Solid Edge part; units mm, degrees
sketch "Sketch1" plane through (0, 0, 0) normal (0, 0, 1) x (1, 0, 0)
  circle A0 centre (0, 0) radius 8
extrude "Protrusion1" add sketch "Sketch1" along normal blind 10
sketch "Sketch2" plane through (0, 0, 0) normal (0, 0, -1) x (1, 0, 0)
  circle A0 centre (0, 0) radius 5
extrude "Protrusion2" add sketch "Sketch2" along normal blind 55
sketch "Sketch3" plane through (0, 0, -55) normal (0, 0, -1) x (1, 0, 0)
  circle A0 centre (0, 0) radius 4.9997
extrude "Cutout1" cut sketch "Sketch3" against normal blind 32 flip side to cut
chamfer "Chamfer_1" distance 0.75 angle 45 1 edges at (-4.9997, 0, -55)
sketch "Sketch4" plane through (0, 0, 10) normal (0, 0, 1) x (1, 0, 0)
  line L0 (-2.3094, 4) -> (2.3094, 4)
  line L1 (4.6188, 0) -> (2.3094, 4)
  line L2 (2.3094, -4) -> (4.6188, 0)
  line L3 (-2.3094, -4) -> (2.3094, -4)
  line L4 (-4.6188, 0) -> (-2.3094, -4)
  line L5 (-2.3094, 4) -> (-4.6188, 0)
extrude "Cutout2" cut sketch "Sketch4" against normal blind 5
properties part number "116106"
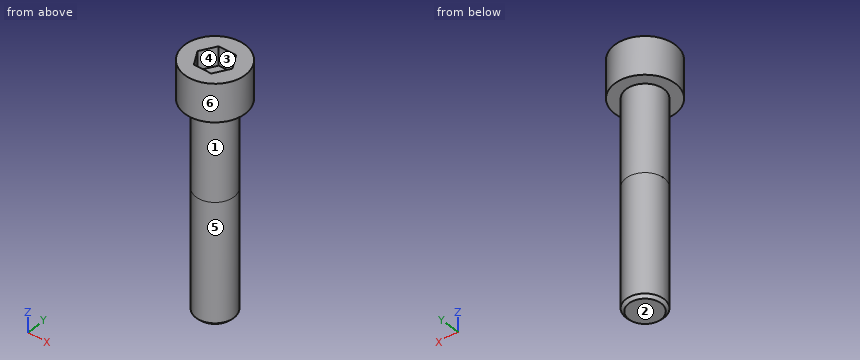
Design review of the part built by this model. Coordinates are the model's own, in mm. Face numbers are marked on the shaded views. A direction names the side the tool comes from. Round coordinates to 2 decimals unless told otherwise and drop trailing zeros. Write each loop counter-clockwise with the first axis right and the second up, starting at its lowest first coordinate (ties: lowest second). Pieces come first, ordered by that corner, then holes. Notation, with made-up numbers: (-17, -20.5) - (-12, -20.5) arc R7 cw to (-12, -13.5) - close; hole circle Ø9 at (29.5, 17). An arc over 180 degrees is marked (long way). Return JSON: item names as keys, results as strings. Group by question number.
Item 1: Insertion check: P1, Ø3, axis at y = -6, z = -40.5, coming from the +X side; P2, Ø1.5, axis at x = 1.5, z = -28, coming from the +Y side; P3, Ø2, axis at y = -3.5, z = -13, coming from the +X side. Each pin has a flat end and moves straight along its axis. Give the tip position at first contact, or say it passes through.
Item 2: Machinability: for the marked faces 4, 5 and 6, which of the approach directions +Z, -Z, +X, -X, +Y, -Y give a long, thin tool a straight path to every point of the face, cutting with its end or side? Answer none if there is none.
Item 3: We need section B-B on z = -8. Write out the cut boundary in (x, y), and give its area (3 significant figures).
Item 4: We need section C-C on y = 6.75. Write out the cut boundary in (x, z), and give its area (3 significant figures).
Item 5: For probe 1 along Z at (x, y) = (0.75, 3.5); probe 2 along Z at (x, y) = (5.75, -2.5); probe 3 along Y at (x, z) = (-0.25, -13.5), list the stretches that pass through material, from the lowest coordinate up. Write a range as [from, to].
Item 6: The part is to be moulded in two halves that separate along X. For the marked faces 1, 2 and 3, say which applies: pulls with the +X half, pulls with the -X half, needs draft (parallel to the pull), parting line crosses it, or undercut.
Model answer:
{
 "1": {"P1": "stops at x = 2.18", "P2": "stops at y = 4.94", "P3": "stops at x = 4.33"},
 "2": {"face 4": "+Z", "face 5": "-Z", "face 6": "+Z, -Z"},
 "3": {"outline": "circle Ø10 at (0, 0)", "area": "78.5 mm²"},
 "4": {"outline": "(-4.29, 0) - (4.29, 0) - (4.29, 10) - (-4.29, 10) - close", "area": "85.9 mm²"},
 "5": {"probe 1": "z = [-55, 5]", "probe 2": "z = [0, 10]", "probe 3": "y = [-4.99, 4.99]"},
 "6": {"face 1": "parting line crosses it", "face 2": "needs draft", "face 3": "undercut"}
}
